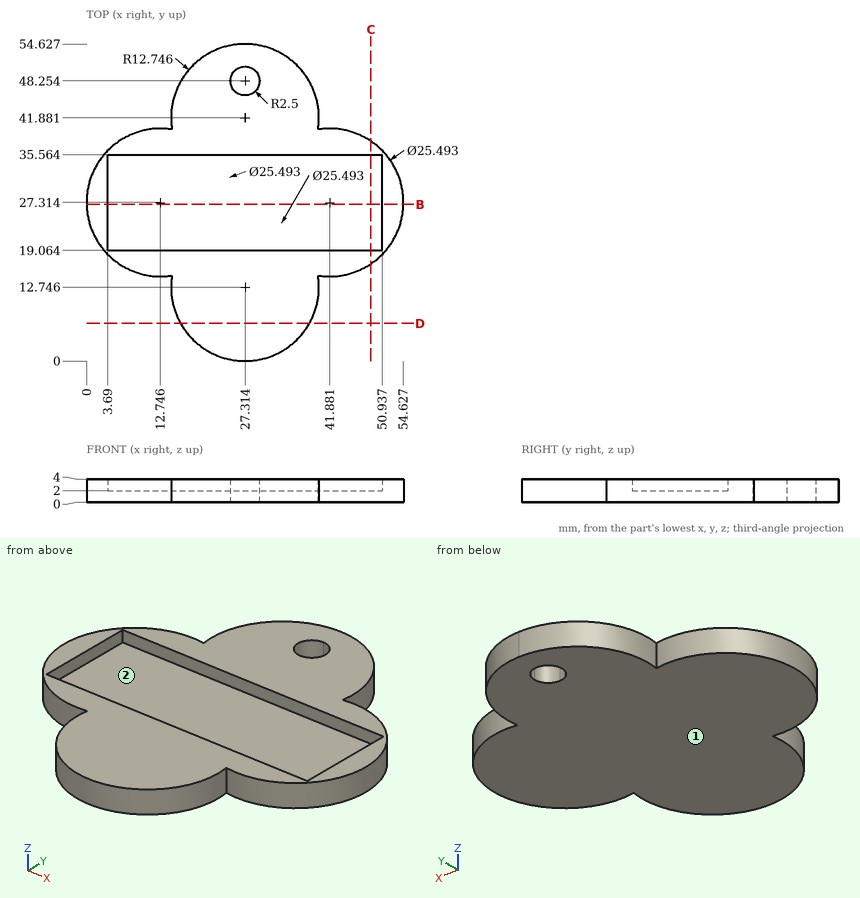
For this review, use the dimensioned drawing (mm, ordinates from the lowest corner) and the shaded views. Give positions to 0.01 mm unless a question says otherwise; leave off trailing zeros. Loops run counter-clockwise (first coordinate to the right, second up) from the corner with the lowest first, then second, coordinate; pieces in that order, holes last. Notation, with made-up numbers: (56, -34.5) - (86, -34.5) arc R20 ccw to (86, 1.5) - close; hole circle Ø6 at (-16.5, 81). An arc over 180 degrees is marked (long way). Write each question's results on one line, items separated by ' | '.
(1) Take a section at C-C (x = 49). Give the boundary of the cut face in (y, z).
Conclusion:
outline: (16.74, 0) - (37.89, 0) - (37.89, 4) - (35.56, 4) - (35.56, 2) - (19.06, 2) - (19.06, 4) - (16.74, 4) - close
(2) Draft analysis for pull direction Y (two halves, no side actions). For the marked faces 1 and 2, state which applies: +Y half, -Y half, draft (parallel to the pull), parting line (faces both ways), or undercut.
Conclusion:
face 1: draft | face 2: undercut
(3) For line 1 along Y through (x, z) = (42.5, 3.8) (1 decimal); line 2 along Z through (x, y) = (31, 26); line 3 along X through (y, z) = (24.5, 3.4) (1 decimal), list the stretches that pass through material, from the lowest coordinate up.
Conclusion:
line 1: 14.6 to 19.1, 35.6 to 40 | line 2: 0 to 2 | line 3: 0.3 to 3.7, 50.9 to 54.3
(4) Take a section at D-D (y = 6.5). Give the boundary of the cut face in (x, z) (1 decimal).
Conclusion:
outline: (16.2, 0) - (38.4, 0) - (38.4, 4) - (16.2, 4) - close
(5) Take a section at B-B (y = 27). Give the boundary of the cut face in (x, z), then the cut area to 3 significant figures.
Conclusion:
outline: (0, 0) - (54.62, 0) - (54.62, 4) - (50.94, 4) - (50.94, 2) - (3.69, 2) - (3.69, 4) - (0, 4) - close | area: 124 mm^2
(6) For pin 1 Ø1 at (x, z) = (26, 3) entering from -Y; pin 2 Ø8.5 at (x, y) = (19, 25) entering from +Z; pin 3 Ø2 at (x, z) = (21, 3.5) entering from +Y, all flat-tipped, find the tip position at first contact; note any pin that passes through.
Conclusion:
pin 1: y = 0.03 | pin 2: z = 2 | pin 3: y = 53.47
